Geometry check sheet. Reference: the model listing, model coordinates, mm. Face numbers are marked on the shaded views. A direction names the side the tool comes from. Round coordinates to 2 decimals unless told otherwise and drop trailing zeros. Loops run counter-clockwise (first coordinate to the right, second up) from the corner with the lowest first, then second, coordinate; pieces in that order, holes last. Notation, with made-up numbers: M 48.5,-10.75 L 90.5,-10.75 A27 ccw 90.5,6.25 Z; hole C -25.75,-4 d2. An arc over 180 degrees is marked long. Use one line per item in the form item = value. Start each with the question number.
1. Cross-section at D-D (y = 1.25). Record the boundary of the cut face in (x, z).
2. Material ranges on line 1 (Z direction, x = 0, y = 2.25); line 2 (Z direction, x = 0, y = -1); line 3 (Y direction, x = 6, z = 4.75), recorded low to high.
3. Cross-section at B-B (x = 0). Record the boundary of the cut face in (y, z).
4. Set-up check for the marked faces 1 and 2: record each of +Z, -Z, +X, -X, +Y, -Y from which the full face is reachable in a straight line by a thin tool's end or side.
5. Cross-section at A-A (z = 5). Record the boundary of the cut face in (x, y).
6. Go/stop test with flat-tipped pins: pin 1 (1.5 mm diameter, centred on x = 5, z = 10, fed in from +Y); pin 2 (3 mm diameter, centred on x = -3, y = 1, fed in from +Z); pin 3 (1 mm diameter, centred on x = -5, z = 6, fed in from -Y); pin 4 (3.5 mm diameter, centred on x = 0, z = 5, fed in from +Y). Record where each tip stops, or that it passes through.
7. Draft check along Z on the marked faces 3, 4 and 5. Enter one of: pulls with the +Z half, pulls with the -Z half, needs draft (parallel to the pull), parting line crosses it, or undercut.
8. Cross-section at C-C (y = 0). Record the boundary of the cut face in (x, z).
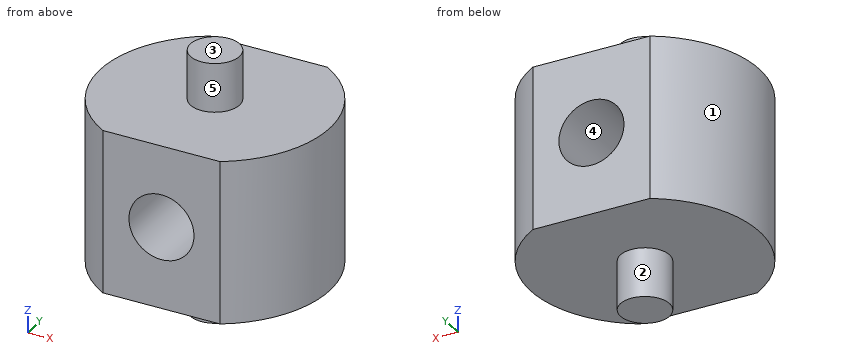
```python
from build123d import *

# Parameters (mm, degrees)
BASE_EXTRUSION_DEPTH = 10
ESQUISSE2_R          = 1.5
BOSS_EXTRU_1_DEPTH   = 3
BOSS_EXTRU_2_START   = 3
ESQUISSE3_R          = 1.5
BOSS_EXTRU_2_DEPTH   = 3
PER_AGE1_D           = 4
PER_AGE1_DEPTH       = 11.99888719
PER_AGE1_TIP         = 1.201721238


with BuildPart() as part:
    # Esquisse1 → Base-Extrusion (new body)
    with BuildSketch(Plane.XY):
        with BuildLine():
            Line((-3.606477028, 5.999443595), (3.606477028, 5.999443595))
            ThreePointArc((3.606477028, 5.999443595), (7, 0), (3.606477028, -5.999443595))
            Line((3.606477028, -5.999443595), (-3.606477028, -5.999443595))
            ThreePointArc((-3.606477028, -5.999443595), (-7, 0), (-3.606477028, 5.999443595))
        make_face()
    extrude(amount=BASE_EXTRUSION_DEPTH)

    # Esquisse2 → Boss.-Extru.1 (add)
    with BuildSketch(Plane.XY.offset(10)):
        Circle(ESQUISSE2_R)
    extrude(amount=BOSS_EXTRU_1_DEPTH)

    # Esquisse3 → Boss.-Extru.2 (add)
    with BuildSketch(Plane(origin=(0, 0, 0), x_dir=(-1, 0, 0), z_dir=(0, 0, -1)).offset(BOSS_EXTRU_2_START)):
        with Locations(Location((0, 0, 0), (0, 0, 180))):
            Circle(ESQUISSE3_R)
    extrude(amount=-BOSS_EXTRU_2_DEPTH)

    # Perçage1
    with Locations(Plane(origin=(0, 5.999443595, 0), x_dir=(-1, 0, 0), z_dir=(0, 1, 0))):
        with Locations((0, 5)):
            Hole(PER_AGE1_D / 2, depth=PER_AGE1_DEPTH)
            with Locations((0, 0, -(PER_AGE1_DEPTH + PER_AGE1_TIP / 2))):  # 118° drill point
                Cone(0, PER_AGE1_D / 2, PER_AGE1_TIP, mode=Mode.SUBTRACT)


solid = part.part
```
Reported:
q1.outline = M -6.89,0 L -0.83,0 L -0.83,-3 L 0.83,-3 L 0.83,0 L 6.89,0 L 6.89,10 L 0.83,10 L 0.83,13 L -0.83,13 L -0.83,10 L -6.89,10 Z; hole C 0,5 d4
q2.line_1 = 0 to 3, 7 to 10
q2.line_2 = -3 to 3, 7 to 13
q2.line_3 = -3.61 to 3.61
q3.outline = M -6,0 L -1.5,0 L -1.5,-3 L 1.5,-3 L 1.5,0 L 6,0 L 6,3 L -6,3 Z; M -6,7 L 6,7 L 6,10 L 1.5,10 L 1.5,13 L -1.5,13 L -1.5,10 L -6,10 Z
q4.face_1 = +Z, -Z, -X
q4.face_2 = -Z
q5.outline = M -3.61,-6 L -2,-6 L -2,6 L -3.61,6 A7 ccw Z; M 2,-6 L 3.61,-6 A7 ccw 3.61,6 L 2,6 Z
q6.pin_1 = 5.56
q6.pin_2 = 10
q6.pin_3 = -5.36
q6.pin_4 = through
q7.face_3 = pulls with the +Z half
q7.face_4 = undercut
q7.face_5 = needs draft
q8.outline = M -7,0 L -1.5,0 L -1.5,-3 L 1.5,-3 L 1.5,0 L 7,0 L 7,10 L 1.5,10 L 1.5,13 L -1.5,13 L -1.5,10 L -7,10 Z; hole C 0,5 d4
